from build123d import *

# Parameters (mm, degrees)
SKETCH2_R           = 1.5
BOSS_EXTRUDE3_DEPTH = 12
SKETCH4_R           = 7.810249676


with BuildPart() as part:
    # Sketch2 → Boss-Extrude3 (new body)
    with BuildSketch(Plane(origin=(0, 0, 0), x_dir=(1, 0, 0), z_dir=(0, 1, 0))):
        with BuildLine():
            ThreePointArc((2.827295528, 49.92), (0, 47.171572875), (-2.827295528, 49.92))
            ThreePointArc((-2.827295528, 49.92), (0, -50), (2.827295528, 49.92))
        make_face()
        with BuildLine():
            ThreePointArc((1.658312395, 2.5), (0, -3), (-1.658312395, 2.5))
            Line((-1.658312395, 2.5), (1.658312395, 2.5))
        make_face(mode=Mode.SUBTRACT)
        with Locations((0, 40)):
            Circle(SKETCH2_R, mode=Mode.SUBTRACT)
    extrude(amount=BOSS_EXTRUDE3_DEPTH)

    # Sketch4 → Cut-Revolve1 (revolve, cut)
    with BuildSketch(Plane.XY):
        with Locations((55, 6)):
            Circle(SKETCH4_R)
    revolve(axis=Axis((0, 0, 0), (0, 1, 0)), mode=Mode.SUBTRACT)


solid = part.part
Model file for the job. Use its own axes, mm. Coordinates: 2 decimals unless noted, no trailing zeros. Write each loop counter-clockwise with the first axis right and the second up, starting at its lowest first coordinate (ties: lowest second). Pieces come first, ordered by that corner, then holes. Notation, with made-up numbers: (-4, 1) -> (53, 1) arc R5 cw to (53, 10) -> close; hole circle Ø6 at (75.5, 9.5). An arc over 180 degrees is marked (long way). One line per item, written item: value. Start each with the question number.
1) Pull direction X, two halves, no side cores. Call faces 1 (the face through (10, 12, -1)), 2 (the face through (0.061, 5.916, -47.172)), 3 (the face through (0, 6, -2.5)): +X half, -X half, draft (parallel to the pull), parting line (faces both ways), or undercut.
2) Probe probe 1 along Z at (x, y) = (0, 7); probe 2 along X at (y, z) = (7, -40). List the from-to ranges inside material, lowest first.
3) Flat gauge pins, fed straight in: pin 1 Ø1.5 at (x, y) = (-27, 3) entering from +Z; pin 2 Ø2 at (y, z) = (3, -25.5) entering from -X; pin 3 Ø6 at (y, z) = (7.5, 7.5) entering from -X. Where does each tip first touch, or does it go through?
4) Slice it at A-A on y = 6.25. Write the cut outline in (x, z).
Answers follow:
1. face 1: draft
1. face 2: undercut
1. face 3: undercut
2. probe 1: -47.17 to -41.5, -38.5 to -2.5, 3 to 47.25
2. probe 2: -25.16 to -1.5, 1.5 to 25.16
3. pin 1: z = 40.08
3. pin 2: x = -41.25
3. pin 3: x = -48.08
4. outline: (-0.34, -47.19) arc R2.83 cw to (0.34, -47.19) arc R47.19 ccw (long way) to start; hole (-1.66, -2.5) -> (1.66, -2.5) arc R3 ccw (long way) to start; hole circle Ø3 at (0, -40)
